Could you check a few things on this model? Use its own coordinates, in mm. Give positions to 0.01 mm unless a question says otherwise; leave off trailing zeros. Write each loop counter-clockwise with the first axis right and the second up, starting at its lowest first coordinate (ties: lowest second). Pieces come first, ordered by that corner, then holes. Notation, with made-up numbers: M 12.25,-26 L 30.25,-26 A9 cw 30.25,-20 Z; hole C -10,86 d11. An arc over 180 degrees is marked long. Answer as a JSON object with one key per item and string values. Group by question number.
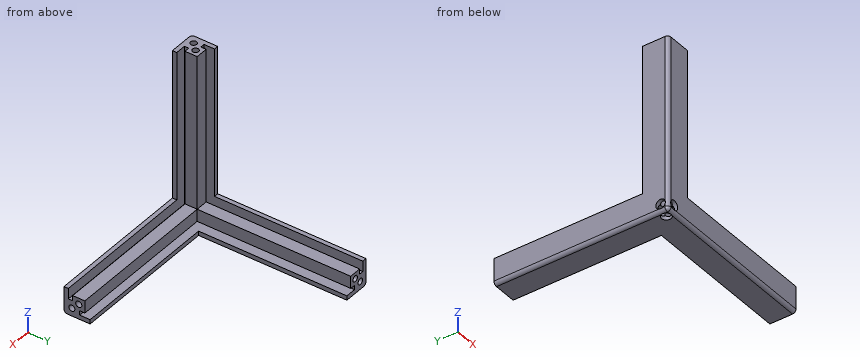
```python
from build123d import *

# Parameters (mm, degrees)
F0_R          = 1.75
F1_DEPTH      = 100
F2_R          = 1.75
F3_DEPTH      = 100
F4_R          = 1.75
F5_DEPTH      = 100
F6_DEPTH      = 3
F7_DEPTH      = 3
F8_DEPTH      = 3
F9_R          = 2.75
F10_DEPTH     = 80
F11_R         = 2.75
F12_DEPTH     = 80
F13_R         = 2.75
F14_DEPTH     = 80
F15_T1_DEPTH  = 103
F15_T3_DEPTH  = 103
F15_T5_DEPTH  = 103
F15_S9_W      = 2
F15_S9_H      = 2
F15_T10_DEPTH = 2
F16_R         = 1.75
F17_DEPTH     = 25
F18_R         = 1.75
F19_DEPTH     = 25
F20_R         = 1.75
F21_DEPTH     = 25


# Not quite as in the source:
# - a fillet or chamfer that OpenCascade refuses, or shapes differently, is made with other operations: its cross-section is extruded or revolved along the edge and cut away or added


with BuildPart() as f1:
    # F0 (on Top) → F1 (new body)
    with BuildSketch(Plane.XY):
        Polygon((2.5, 15), (0, 15), (0, 0), (15, 0), (15, 2.5), (9, 2.5), (9, 5), (12, 5), (12, 12), (5, 12), (5, 9), (2.5, 9), align=None)
        with Locations((4.5, 4.5)):
            Circle(F0_R, mode=Mode.SUBTRACT)
    extrude(amount=F1_DEPTH)

    # F2 (on Right) → F3 (join)
    with BuildSketch(Plane.YZ):
        Polygon((2.5, 15), (0, 15), (0, 0), (15, 0), (15, 2.5), (9, 2.5), (9, 5), (12, 5), (12, 12), (5, 12), (5, 9), (2.5, 9), align=None)
        with Locations((4.5, 4.5)):
            Circle(F2_R, mode=Mode.SUBTRACT)
    extrude(amount=F3_DEPTH)

    # F4 (on Front) → F5 (join)
    with BuildSketch(Plane.XZ):
        Polygon((2.5, 15), (0, 15), (0, 0), (15, 0), (15, 2.5), (9, 2.5), (9, 5), (12, 5), (12, 12), (5, 12), (5, 9), (2.5, 9), align=None)
        with Locations((4.5, 4.5)):
            Circle(F4_R, mode=Mode.SUBTRACT)
    extrude(amount=-F5_DEPTH)

    # F6 (cut): a face of the model
    f6_faces = [f1.faces().sort_by_distance(p)[0] for p in [
        (3.75, 12, 10.5),
    ]]
    extrude(f6_faces, amount=-F6_DEPTH, mode=Mode.SUBTRACT)

    # F7 (cut): a face of the model
    f7_faces = [f1.faces().sort_by_distance(p)[0] for p in [
        (12, 3.75, 10.5),
    ]]
    extrude(f7_faces, amount=-F7_DEPTH, mode=Mode.SUBTRACT)

    # F8 (cut): a face of the model
    f8_faces = [f1.faces().sort_by_distance(p)[0] for p in [
        (12, 10.5, 3.75),
    ]]
    extrude(f8_faces, amount=-F8_DEPTH, mode=Mode.SUBTRACT)

    # F9 (on face) → F10 (cut)
    with BuildSketch(Plane(origin=(0, 0, 0), x_dir=(0, -1, 0), z_dir=(-1, 0, 0))):
        with Locations((-4.5, 4.5)):
            Circle(F9_R)
    extrude(amount=-F10_DEPTH, mode=Mode.SUBTRACT)

    # F11 (on face) → F12 (cut)
    with BuildSketch(Plane(origin=(0, 0, 0), x_dir=(1, 0, 0), z_dir=(0, 0, -1))):
        with Locations((4.5, -4.5)):
            Circle(F11_R)
    extrude(amount=-F12_DEPTH, mode=Mode.SUBTRACT)

    # F13 (on face) → F14 (cut)
    with BuildSketch(Plane.XZ):
        with Locations((4.5, 4.5)):
            Circle(F13_R)
    extrude(amount=-F14_DEPTH, mode=Mode.SUBTRACT)

    # F15: fillet of radius 2 on 3 edges, made by hand

    # F15_s2 → F15_t1 (cut)
    with BuildSketch(Plane.XZ.offset(-105)):
        with BuildLine():
            ThreePointArc((2, 0), (0.5857864376, 0.5857864376), (0, 2))
            Line((0, 2), (0, 0))
            Line((0, 0), (2, 0))
        make_face()
    extrude(amount=F15_T1_DEPTH, mode=Mode.SUBTRACT)

    # F15_s4 → F15_t3 (cut)
    with BuildSketch(Plane.YZ.offset(2)):
        with BuildLine():
            ThreePointArc((2, 0), (0.5857864376, 0.5857864376), (0, 2))
            Line((0, 2), (0, 0))
            Line((0, 0), (2, 0))
        make_face()
    extrude(amount=F15_T3_DEPTH, mode=Mode.SUBTRACT)

    # F15_s6 → F15_t5 (cut)
    with BuildSketch(Plane.XY.offset(2)):
        with BuildLine():
            ThreePointArc((2, 0), (0.5857864376, 0.5857864376), (0, 2))
            Line((0, 2), (0, 0))
            Line((0, 0), (2, 0))
        make_face()
    extrude(amount=F15_T5_DEPTH, mode=Mode.SUBTRACT)


with BuildPart() as f15_tool8:
    # F15_s9 → F15_t10 (new body)
    with BuildSketch(Plane.XY.offset(2)):
        with Locations((1, 1)):
            Rectangle(F15_S9_W, F15_S9_H)
    extrude(amount=-F15_T10_DEPTH)

    # F15_s11 → F15_t12 (revolve, cut)
    with BuildSketch(Plane(origin=(2, 2, 2), x_dir=(0.7071067812, 0.7071067812, 0), z_dir=(-0.7071067812, 0.7071067812, 0))):
        with BuildLine():
            ThreePointArc((0, -2), (2, 0), (0, 2))
            Line((0, 2), (0, -2))
        make_face()
    revolve(axis=Axis((2, 2, 2), (0, 0, -1)), mode=Mode.SUBTRACT)


with BuildPart() as f1_1:
    add(f1.part)

    # F15_t7: cut F15_tool8
    add(f15_tool8.part, mode=Mode.SUBTRACT)

    # F16 (on face) → F17 (cut)
    with BuildSketch(Plane.YZ.offset(100)):
        with Locations((8.5, 8.5)):
            Circle(F16_R)
    extrude(amount=-F17_DEPTH, mode=Mode.SUBTRACT)

    # F18 (on face) → F19 (cut)
    with BuildSketch(Plane.XY.offset(100)):
        with Locations((8.5, 8.5)):
            Circle(F18_R)
    extrude(amount=-F19_DEPTH, mode=Mode.SUBTRACT)

    # F20 (on face) → F21 (cut)
    with BuildSketch(Plane(origin=(0, 100, 0), x_dir=(-1, 0, 0), z_dir=(0, 1, 0))):
        with Locations((-8.5, 8.5)):
            Circle(F20_R)
    extrude(amount=-F21_DEPTH, mode=Mode.SUBTRACT)


solid = f1_1.part
```
1) Please list where these lines run through material, in increasing order: line 1 along Y through (x, z) = (8.5, 85.25); line 2 along X through (y, z) = (25, 4.5); line 3 along Y through (x, z) = (11, 91.5). Write a range as from..to.
2) If we section it at A-A, the plane y = 30: List the corners of the cut face in (x, z) for me.
3) I'm going to push flat-ended pins straight in: pin 1 (4 mm diameter, centred on x = 4.5, z = 4.5, fed in from -Y); pin 2 (3 mm diameter, centred on x = 1.5, z = 51, fed in from +Y); pin 3 (1 mm diameter, centred on x = 8.5, z = 8.5, fed in from +Y); pin 4 (12 mm diameter, centred on x = 38.5, y = 25.5, fed in from -Z). Where does each tip first touch, or does it pass through?
4) If we section it at C-C, the plane y = 91: List the corners of the cut face in (x, z) for me.
Taken from the geometry:
{
 "1": {"line 1": "0..6.75, 10.25..12", "line 2": "0..1.75, 7.25..9", "line 3": "0..2.5, 5..12"},
 "2": {"outline": "M 0,2 A2 ccw 2,0 L 15,0 L 15,2.5 L 9,2.5 L 9,5 L 12,5 L 12,12 L 5,12 L 5,9 L 2.5,9 L 2.5,15 L 0,15 Z; hole C 4.5,4.5 d5.5"},
 "3": {"pin 1": "y = 80", "pin 2": "y = 15", "pin 3": "y = 75", "pin 4": "through"},
 "4": {"outline": "M 0,2 A2 ccw 2,0 L 15,0 L 15,2.5 L 9,2.5 L 9,5 L 12,5 L 12,12 L 5,12 L 5,9 L 2.5,9 L 2.5,15 L 0,15 Z; hole C 4.5,4.5 d3.5; hole C 8.5,8.5 d3.5"}
}
